```python
from build123d import *

# Parameters (mm, degrees)
SKETCH3_W                 = 75
SKETCH3_H                 = 254
BOSS_EXTRUDE2_DEPTH       = 35
SHELL2_T                  = -6
CUT_EXTRUDE1_DEPTH        = 2
CUT_EXTRUDE2_DEPTH        = 137.000919115
SKETCH6_W                 = 14
SKETCH6_H                 = 184
CUT_EXTRUDE3_DEPTH        = 152.58825812
FILLET1_R                 = 10
FILLET2_R                 = 5
SKETCH12_W                = 57.5
SKETCH12_H                = 8
BOSS_EXTRUDE4_DEPTH       = 35
FILLET5_R                 = 10
FILLET6_R                 = 15
M8X1_0_TAPPED_HOLE1_D     = 7
M8X1_0_TAPPED_HOLE1_DEPTH = 8
M8X1_0_TAPPED_HOLE1_TIP   = 2.103012167
SKETCH16_R                = 24
CUT_EXTRUDE4_DEPTH        = 91
BOSS_EXTRUDE5_DEPTH       = 6
CUT_EXTRUDE5_DEPTH        = 29


with BuildPart() as part:
    # Sketch3 → Boss-Extrude2 (new body)
    with BuildSketch(Plane(origin=(0, 0, 0), x_dir=(0, 0, -1), z_dir=(1, 0, 0))):
        Rectangle(SKETCH3_W, SKETCH3_H)
    extrude(amount=BOSS_EXTRUDE2_DEPTH)

    # Shell2
    shell2_openings = [part.faces().sort_by_distance(p)[0] for p in [
        (35, 0, 0),
    ]]
    offset(amount=SHELL2_T, openings=shell2_openings, kind=Kind.INTERSECTION)

    # Sketch4 → Cut-Extrude1 (cut)
    with BuildSketch(Plane(origin=(6, 0, 0), x_dir=(0, 0, -1), z_dir=(1, 0, 0))):
        with BuildLine():
            Line((12.9, -5.439669108), (12.9, 5.439669108))
            ThreePointArc((12.9, 5.439669108), (0.363761531, 13.9952734), (-12.6, 6.102458521))
            Line((-12.6, 6.102458521), (-12.6, -6.102458521))
            ThreePointArc((-12.6, -6.102458521), (0.363761531, -13.9952734), (12.9, -5.439669108))
        make_face()
    cut_extrude1 = extrude(amount=-CUT_EXTRUDE1_DEPTH, mode=Mode.SUBTRACT)

    # Sketch5 → Cut-Extrude2 (cut, through all)
    with BuildSketch(Plane(origin=(4, 0, 0), x_dir=(0, 0, -1), z_dir=(1, 0, 0))):
        with BuildLine():
            Line((9.9, -4.794788838), (9.9, 4.794788838))
            ThreePointArc((9.9, 4.794788838), (0, 11), (-9.9, 4.794788838))
            Line((-9.9, 4.794788838), (-9.9, -4.794788838))
            ThreePointArc((-9.9, -4.794788838), (0, -11), (9.9, -4.794788838))
        make_face()
    cut_extrude2 = extrude(amount=-CUT_EXTRUDE2_DEPTH, mode=Mode.SUBTRACT)

    # Sketch6 → Cut-Extrude3 (cut, through all)
    with BuildSketch(Plane.XY.offset(37.5)):
        with Locations((17.5, 0)):
            Rectangle(SKETCH6_W, SKETCH6_H)
    extrude(amount=-CUT_EXTRUDE3_DEPTH, mode=Mode.SUBTRACT)

    # Fillet1
    fillet1_edges = [part.edges().sort_by_distance(p)[0] for p in [
        (17.5, -127, -37.5),
        (17.5, -127, 37.5),
        (17.5, 127, 37.5),
        (17.5, 127, -37.5),
    ]]
    fillet(fillet1_edges, radius=FILLET1_R)

    # Fillet2
    fillet2_edges = [part.edges().sort_by_distance(p)[0] for p in [
        (20.5, -121, -31.5),
        (20.5, 121, -31.5),
        (20.5, 121, 31.5),
        (20.5, -121, 31.5),
    ]]
    fillet(fillet2_edges, radius=FILLET2_R)

    # Sketch12 → Boss-Extrude4 (add)
    with BuildSketch(Plane(origin=(35, 0, 0), x_dir=(0, 0, -1), z_dir=(1, 0, 0))):
        with Locations((-66.25, -105)):
            Rectangle(SKETCH12_W, SKETCH12_H)
    extrude(amount=-BOSS_EXTRUDE4_DEPTH)

    # Fillet5
    # the kernel refuses this fillet: 10 mm, written as the material it adds along each edge
    with BuildSketch(Plane(origin=(35, -109, 37.5), x_dir=(0, -0.9999844906159053, -0.0055694279462415305), z_dir=(-1, 0, 0))) as fillet5_piece_1:
        with BuildLine():
            CenterArc((9.944708969, 9.955289483), FILLET5_R, 180.319106365, 84.260829523)
            Line((-0.055135937, 9.899595203), (-1.055120428, 9.894025775))
            Line((-1.055120428, 9.894025775), (-0.999984491, -0.005569428))
            Line((-0.999984491, -0.005569428), (0.005569428, -0.999984491))
            ThreePointArc((0.005569428, -0.999984491), (8.005445353, -0.955429067), (8.905682648, -0.995528948))
            Line((8.905682648, -0.995528948), (9.000139587, 0))
        make_face()
    extrude(amount=35)
    with BuildSketch(Plane(origin=(35, -101, 37.5), x_dir=(0, 1, 0), z_dir=(-1, 0, 0))) as fillet5_piece_2_section:
        with BuildLine():
            CenterArc((FILLET5_R, -FILLET5_R), FILLET5_R, 90, 90)
            Line((0, -FILLET5_R), (0, 0))
            Line((0, 0), (FILLET5_R, 0))
        make_face()
    fillet5_piece_2 = extrude(amount=35, mode=Mode.PRIVATE)
    fillet5_piece_2 = split(fillet5_piece_2, bisect_by=Plane(origin=(29.75, -92, 37.408860849), z_dir=(0, 1, 0)), keep=Keep.TOP, mode=Mode.PRIVATE)
    fillet5_piece_2 = split(fillet5_piece_2, bisect_by=Plane(origin=(24.5, -91.519267155, 37.408860849), z_dir=(1, 0, 0)), keep=Keep.TOP, mode=Mode.PRIVATE)
    add(fillet5_piece_2)
    with BuildSketch(Plane(origin=(35, -101, 37.5), x_dir=(0, 1, 0), z_dir=(-1, 0, 0))) as fillet5_piece_3_section:
        with BuildLine():
            CenterArc((FILLET5_R, -FILLET5_R), FILLET5_R, 90, 90)
            Line((0, -FILLET5_R), (0, 0))
            Line((0, 0), (FILLET5_R, 0))
        make_face()
    fillet5_piece_3 = extrude(amount=35, mode=Mode.PRIVATE)
    fillet5_piece_3 = split(fillet5_piece_3, bisect_by=Plane(origin=(29.75, -92, 39.784135406), z_dir=(0, -1, 0)), keep=Keep.TOP, mode=Mode.PRIVATE)
    fillet5_piece_3 = split(fillet5_piece_3, bisect_by=Plane(origin=(24.5, -98.797900168, 39.784135406), z_dir=(1, 0, 0)), keep=Keep.TOP, mode=Mode.PRIVATE)
    add(fillet5_piece_3)
    with BuildSketch(Plane(origin=(35, -101, 37.5), x_dir=(0, 1, 0), z_dir=(-1, 0, 0))) as fillet5_piece_4_section:
        with BuildLine():
            CenterArc((FILLET5_R, -FILLET5_R), FILLET5_R, 90, 90)
            Line((0, -FILLET5_R), (0, 0))
            Line((0, 0), (FILLET5_R, 0))
        make_face()
    fillet5_piece_4 = extrude(amount=35, mode=Mode.PRIVATE)
    fillet5_piece_4 = split(fillet5_piece_4, bisect_by=Plane(origin=(10.5, -98.797900168, 39.784135406), z_dir=(1, 0, 0)), keep=Keep.TOP, mode=Mode.PRIVATE)
    fillet5_piece_4 = split(fillet5_piece_4, bisect_by=Plane(origin=(17.5, -92, 39.784135406), z_dir=(0, -1, 0)), keep=Keep.TOP, mode=Mode.PRIVATE)
    fillet5_piece_4 = split(fillet5_piece_4, bisect_by=Plane(origin=(24.5, -98.797900168, 39.784135406), z_dir=(-1, 0, 0)), keep=Keep.TOP, mode=Mode.PRIVATE)
    add(fillet5_piece_4)
    with BuildSketch(Plane(origin=(35, -101, 37.5), x_dir=(0, 1, 0), z_dir=(-1, 0, 0))) as fillet5_piece_5_section:
        with BuildLine():
            CenterArc((FILLET5_R, -FILLET5_R), FILLET5_R, 90, 90)
            Line((0, -FILLET5_R), (0, 0))
            Line((0, 0), (FILLET5_R, 0))
        make_face()
    fillet5_piece_5 = extrude(amount=35, mode=Mode.PRIVATE)
    fillet5_piece_5 = split(fillet5_piece_5, bisect_by=Plane(origin=(10.5, -91.519267155, 37.408860849), z_dir=(-1, 0, 0)), keep=Keep.TOP, mode=Mode.PRIVATE)
    fillet5_piece_5 = split(fillet5_piece_5, bisect_by=Plane(origin=(5.25, -92, 37.408860849), z_dir=(0, 1, 0)), keep=Keep.TOP, mode=Mode.PRIVATE)
    add(fillet5_piece_5)
    with BuildSketch(Plane(origin=(35, -101, 37.5), x_dir=(0, 1, 0), z_dir=(-1, 0, 0))) as fillet5_piece_6_section:
        with BuildLine():
            CenterArc((FILLET5_R, -FILLET5_R), FILLET5_R, 90, 90)
            Line((0, -FILLET5_R), (0, 0))
            Line((0, 0), (FILLET5_R, 0))
        make_face()
    fillet5_piece_6 = extrude(amount=35, mode=Mode.PRIVATE)
    fillet5_piece_6 = split(fillet5_piece_6, bisect_by=Plane(origin=(10.5, -98.797900168, 39.784135406), z_dir=(-1, 0, 0)), keep=Keep.TOP, mode=Mode.PRIVATE)
    fillet5_piece_6 = split(fillet5_piece_6, bisect_by=Plane(origin=(5.25, -92, 39.784135406), z_dir=(0, -1, 0)), keep=Keep.TOP, mode=Mode.PRIVATE)
    add(fillet5_piece_6)

    # Fillet6
    fillet6_edges = [part.edges().sort_by_distance(p)[0] for p in [
        (35, -105, 95),
        (0, -105, 95),
    ]]
    fillet(fillet6_edges, radius=FILLET6_R)

    # M8x1.0 Tapped Hole1
    with Locations(Plane(origin=(17.5, -101, 62), x_dir=(0, 0, 1), z_dir=(0, 1, 0))):
        with Locations((0, 0)):
            Hole(M8X1_0_TAPPED_HOLE1_D / 2, depth=M8X1_0_TAPPED_HOLE1_DEPTH)
            with Locations((0, 0, -(M8X1_0_TAPPED_HOLE1_DEPTH + M8X1_0_TAPPED_HOLE1_TIP / 2))):  # 118° drill point
                Cone(0, M8X1_0_TAPPED_HOLE1_D / 2, M8X1_0_TAPPED_HOLE1_TIP, mode=Mode.SUBTRACT)

    # Sketch16 → Cut-Extrude4 (cut)
    with BuildSketch(Plane(origin=(0, -101, 0), x_dir=(1, 0, 0), z_dir=(0, 1, 0))):
        with Locations((17.5, -62)):
            Circle(SKETCH16_R)
    extrude(amount=CUT_EXTRUDE4_DEPTH, mode=Mode.SUBTRACT)

    # Sketch17 → Boss-Extrude5 (add)
    with BuildSketch(Plane(origin=(35, 0, 0), x_dir=(0, 0, -1), z_dir=(1, 0, 0))):
        with BuildLine():
            Line((-26.806920407, -127), (28.193079593, -127))
            ThreePointArc((28.193079593, -127), (35.264147405, -124.071067812), (38.193079593, -117))
            Line((38.193079593, -117), (38.193079593, 117))
            ThreePointArc((38.193079593, 117), (35.264147405, 124.071067812), (28.193079593, 127))
            Line((28.193079593, 127), (-26.806920527, 127))
            ThreePointArc((-26.806920527, 127), (-33.878742431, 124.070313639), (-36.806920299, 116.997866992))
            Line((-36.806920299, 116.997866992), (-36.756795058, -117.999997222))
            ThreePointArc((-36.756795058, -117.999997222), (-33.515125375, -124.416197551), (-26.806920407, -127))
        make_face()
    extrude(amount=-BOSS_EXTRUDE5_DEPTH)

    # Mirror1: Cut-Extrude1, Cut-Extrude2 across plane
    add(cut_extrude1.mirror(Plane.ZY.offset(-17.5)), mode=Mode.SUBTRACT)
    add(cut_extrude2.mirror(Plane.ZY.offset(-17.5)), mode=Mode.SUBTRACT)

    # Sketch18 → Cut-Extrude5 (cut)
    with BuildSketch(Plane.ZY):
        with BuildLine():
            ThreePointArc((31.5, 117), (30.328427125, 119.828427125), (27.5, 121))
            Line((27.5, 121), (-27.5, 121))
            ThreePointArc((-27.5, 121), (-30.328427125, 119.828427125), (-31.5, 117))
            Line((-31.5, 117), (-31.5, -117))
            ThreePointArc((-31.5, -117), (-30.328427125, -119.828427125), (-27.5, -121))
            Line((-27.5, -121), (27.5, -121))
            ThreePointArc((27.5, -121), (30.328427125, -119.828427125), (31.5, -117))
            Line((31.5, -117), (31.5, 117))
        make_face()
        with BuildLine():
            Line((-9.9, -4.794788838), (-9.9, 4.794788838))
            ThreePointArc((-9.9, 4.794788838), (0, 11), (9.9, 4.794788838))
            Line((9.9, 4.794788838), (9.9, -4.794788838))
            ThreePointArc((9.9, -4.794788838), (0, -11), (-9.9, -4.794788838))
        make_face(mode=Mode.SUBTRACT)
    extrude(amount=-CUT_EXTRUDE5_DEPTH, mode=Mode.SUBTRACT)


solid = part.part
```
The model under review builds one solid part; all positions refer to its coordinate system, in mm. A direction names the side the tool comes from. Round coordinates to 2 decimals unless told otherwise and drop trailing zeros. Loops run counter-clockwise (first coordinate to the right, second up) from the corner with the lowest first, then second, coordinate; pieces in that order, holes last. Notation, with made-up numbers: (-38.75, -17) - (-20.75, -17) arc R13 ccw to (-20.75, 4) - close; hole circle Ø2 at (-38, -16.5). An arc over 180 degrees is marked (long way). Use a Markdown table: item, result. Add a question column.
Q1. Add section C-C (y = 72). State the section outline as (x, z) points, plus the area to 3 significant figures.
Q2. Add section B-B (z = 62). State the section outline as (x, y) points, plus the area to 3 significant figures.
Q3. Add section D-D (z = -23). State the section outline as (x, y) points.
Q4. Insertion check: pin 1 Ø1 at (x, y) = (8, -25.5) entering from -Z; pin 2 Ø19 at (y, z) = (19.5, 8) entering from -X; pin 3 Ø1.8 at (x, z) = (18, 34.5) entering from -Y. Each pin has a flat end and moves straight along its axis. Give the tip position at first contact, or say it passes through.
Q5. Add section A-A (x = 17.5). State how many separate pieces and enclosed holes the cut face has, plus the area to 3 significant figures.
Q6. Machinability: for faces 4 (the face through (29.986, 13.988, -0.588)), 5 (the face through (18, -109, 72)), 6 (the face through (24.5, -1, -34)), 7 (the face through (17, -127, 0)), which of the approach directions +Z, -Z, +X, -X, +Y, -Y give a long, thin tool a straight path to every point of the face, cutting with its end or side? Answer none if there is none.
Q7. The part is to be moulded in two halves that separate along X. For faces 1 (the face through (17, 127, 0)), 2 (the face through (24.5, -1, 34)), 3 (the face through (29, 1, -38)), say which applies: pulls with the +X half, pulls with the -X half, needs draft (parallel to the pull), parting line crosses it, or undercut.
Q8. For probe 1 along Z at (x, y) = (17.5, -106.5); probe 2 along Z at (x, y) = (8.5, -11); probe 3 along X at (y, z) = (-105, 62), list the stretches that pass through material, from the lowest coordinate up.
Worked answers:
| question | item | result |
|---|---|---|
| 1 | outline | (0, -37.5) - (10.5, -37.5) - (10.5, -31.5) - (0, -31.5) - close; (0, 31.5) - (10.5, 31.5) - (10.5, 37.5) - (0, 37.5) - close; (24.5, -37.5) - (29, -37.5) - (29, -38.19) - (35, -38.19) - (35, 37.5) - (24.5, 37.5) - (24.5, 31.5) - (29, 31.5) - (29, -31.5) - (24.5, -31.5) - close |
| 1 | area | 634 mm² |
| 2 | outline | (0, -109) - (14, -109) - (14, -101) - (0, -101) - close; (21, -109) - (35, -109) - (35, -101) - (21, -101) - close |
| 2 | area | 224 mm² |
| 3 | outline | (0, -127) - (35, -127) - (35, 127) - (0, 127) - (0, 121) - (29, 121) - (29, -121) - (0, -121) - close |
| 4 | pin 1 | z = -37.5 |
| 4 | pin 2 | x = 29 |
| 4 | pin 3 | y = -124.92 |
| 5 | separate pieces | 3 |
| 5 | enclosed holes | 0 |
| 5 | area | 1,950 mm² |
| 6 | face 4 | -X |
| 6 | face 5 | +Z, +X, -X, -Y |
| 6 | face 6 | +Z, -Z |
| 6 | face 7 | +Z, -Z, +X, -X, -Y |
| 7 | face 1 | needs draft |
| 7 | face 2 | undercut |
| 7 | face 3 | pulls with the -X half |
| 8 | probe 1 | -37.5 to -31.5, 31.5 to 58.5, 65.5 to 95 |
| 8 | probe 2 | -37.5 to -31.5, 31.5 to 37.5 |
| 8 | probe 3 | 0 to 14, 21 to 35 |
